CAD build for the part. Positions are in the model's coordinates, mm. Face numbers are marked on the shaded views. A direction names the side the tool comes from. Round coordinates to 2 decimals unless told otherwise and drop trailing zeros. Loops run counter-clockwise (first coordinate to the right, second up) from the corner with the lowest first, then second, coordinate; pieces in that order, holes last. Notation, with made-up numbers: M -8.75,85.25 L 40.25,85.25 A28 cw 40.25,118.25 Z; hole C 25,-2 d1. An arc over 180 degrees is marked long. Use one line per item in the form item = value.
from build123d import *

# Parameters (mm, degrees)
EXTRUDE_1_DEPTH     = 40
FILLET_1_R          = 1
SKETCH_3_R          = 1.6
CUT_EXTRUDE_1_DEPTH = 40
FILLET_2_R          = 3
FILLET_3_RADIUS     = 20
FILLET_3_LENGTH     = 2
SKETCH_4_R          = 1.6
CUT_EXTRUDE_2_DEPTH = 40


with BuildPart() as part:
    # 草图1 → 凸台-拉伸1 (new body)
    with BuildSketch(Plane.XY):
        Polygon((0, 0), (0, 47.5), (2, 47.5), (2, 2), (41, 2), (41, 0), align=None)
    extrude(amount=EXTRUDE_1_DEPTH)

    # 圆角1
    fillet_1_edges = [part.edges().sort_by_distance(p)[0] for p in [
        (0, 0, 20),
        (2, 2, 20),
    ]]
    fillet(fillet_1_edges, radius=FILLET_1_R)

    # 草图3 → 切除-拉伸1 (cut)
    with BuildSketch(Plane.XZ):
        with Locations((33, 35)):
            Circle(SKETCH_3_R)
        with Locations((33, 5)):
            Circle(SKETCH_3_R)
        with Locations((9, 35)):
            Circle(SKETCH_3_R)
        with Locations((9, 5)):
            Circle(SKETCH_3_R)
    extrude(amount=-CUT_EXTRUDE_1_DEPTH, mode=Mode.SUBTRACT)

    # 圆角2
    fillet_2_edges = [part.edges().sort_by_distance(p)[0] for p in [
        (41, 1, 0),
        (41, 1, 40),
    ]]
    fillet(fillet_2_edges, radius=FILLET_2_R)

    # 圆角3: full round fillet: the end face becomes a half cylinder, R = half its width
    fillet_3_face = Plane((1, 47.5, 20), x_dir=(1, 0, 0), z_dir=(0, 1, 0))  # on the end face: x along it, z out of the body
    fillet_3_slab = fillet_3_face.offset(-FILLET_3_RADIUS / 2) * Box(FILLET_3_LENGTH, 2 * FILLET_3_RADIUS, FILLET_3_RADIUS, mode=Mode.PRIVATE)  # the body's end, R deep
    fillet_3_round = Plane((1, 27.5, 20), x_dir=(0, 1, 0), z_dir=(1, 0, 0)) * Cylinder(FILLET_3_RADIUS, FILLET_3_LENGTH, mode=Mode.PRIVATE)  # its axis R under the face
    add(fillet_3_slab - fillet_3_round, mode=Mode.SUBTRACT)

    # 草图4 → 切除-拉伸2 (cut)
    with BuildSketch(Plane.ZY):
        with Locations((35.5, 26.5)):
            Circle(SKETCH_4_R)
        with Locations((27.75, 13.076606241)):
            Circle(SKETCH_4_R)
        with Locations((12.25, 13.076606241)):
            Circle(SKETCH_4_R)
        with Locations((4.5, 26.5)):
            Circle(SKETCH_4_R)
        with Locations((12.25, 39.923393759)):
            Circle(SKETCH_4_R)
        with Locations((27.75, 39.923393759)):
            Circle(SKETCH_4_R)
        with BuildLine():
            Line((13.5, 19.5), (13.5, 33.5))
            ThreePointArc((13.5, 33.5), (20, 40), (26.5, 33.5))
            Line((26.5, 33.5), (26.5, 19.5))
            ThreePointArc((26.5, 19.5), (20, 13), (13.5, 19.5))
        make_face()
    extrude(amount=-CUT_EXTRUDE_2_DEPTH, mode=Mode.SUBTRACT)


solid = part.part
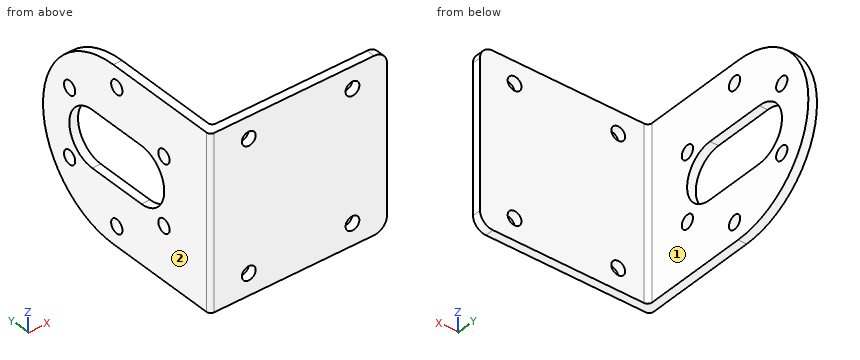
1. Cut at B-B on x = 33. Write the cut outline in (y, z).
Completed:
outline = M 0,0 L 2,0 L 2,3.4 L 0,3.4 Z; M 0,6.6 L 2,6.6 L 2,33.4 L 0,33.4 Z; M 0,36.6 L 2,36.6 L 2,40 L 0,40 Z
2. Cut at D-D on x = 23.5. Write the cut outline in (y, z), and give its area (3 significant figures).
Completed:
outline = M 0,0 L 2,0 L 2,40 L 0,40 Z
area = 80.0 mm2
3. Tool access for the marked faces 1 and 2: list every direction of +Z, -Z, +X, -X, +Y, -Y with a clear straight run to the whole face (end or side of a thin tool).
Completed:
face_1 = +Z, -Z, +X, +Y
face_2 = +Z, -Z, -X, +Y, -Y
4. Cut at A-A on z = 20. Write the cut outline in (x, y), and give its area (3 significant figures).
Completed:
outline = M 0,1 A1 ccw 1,0 L 41,0 L 41,2 L 3,2 A1 cw 2,3 L 2,13 L 0,13 Z; M 0,40 L 2,40 L 2,47.5 L 0,47.5 Z
area = 119 mm2
5. Cut at C-C on z = 12.25. Write the cut outline in (x, y), and give its area (3 significant figures).
Completed:
outline = M 0,1 A1 ccw 1,0 L 41,0 L 41,2 L 3,2 A1 cw 2,3 L 2,11.48 L 0,11.48 Z; M 0,14.68 L 2,14.68 L 2,38.32 L 0,38.32 Z; M 0,41.52 L 2,41.52 L 2,45.94 L 0,45.94 Z
area = 157 mm2
6. Probe line 1 along Y through (x, z) = (14.5, 37.5). List the from-to ranges inside material, lowest first. Write a range as from..to.
Completed:
line_1 = 0..2
7. Drop flat-ended pins along their axis: P1, Ø2.5, axis at y = 13.08, z = 12.25, coming from the -X side; P2, Ø3.5, axis at x = 9, z = 5, coming from the +Y side; P3, Ø1, axis at y = 31.5, z = 35.5, coming from the +X side. Give the stop position or say it passes through.
Completed:
P1 = through
P2 = 2
P3 = 2
